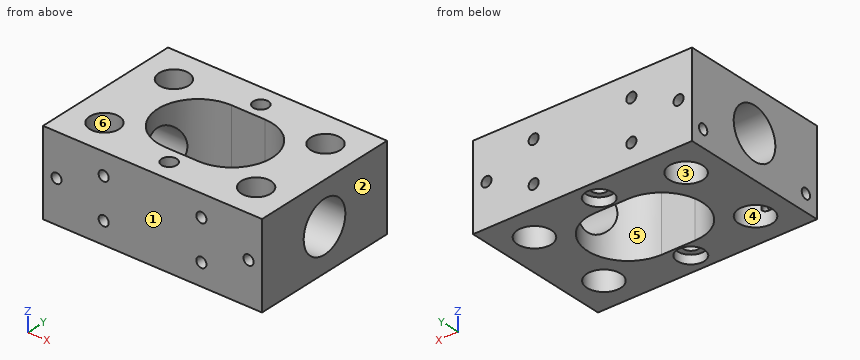
from build123d import *

# Parameters (mm, degrees)
SCHIZZO1_W                                           = 65
SCHIZZO1_H                                           = 45
ESTRUSIONE_ESTRUSIONE1_DEPTH                         = 25
SCHIZZO2_R                                           = 7.5
TAGLIO_ESTRUSIONE1_DEPTH                             = 83.915619759
FORO_LAMATO_PER_VITE_M4_A_TESTA_CILINDRI_D           = 4.5
FORO_LAMATO_PER_VITE_M4_A_TESTA_CILINDRI_CBORE_D     = 8
FORO_LAMATO_PER_VITE_M4_A_TESTA_CILINDRI_CBORE_DEPTH = 2.6
TAGLIO_ESTRUSIONE4_DEPTH                             = 83.915619759
SCHIZZO15_R                                          = 4.4
TAGLIO_ESTRUSIONE5_DEPTH                             = 6
SCHIZZO16_R                                          = 3
TAGLIO_ESTRUSIONE6_DEPTH                             = 82.308056285
SCHIZZO17_R                                          = 5
TAGLIO_ESTRUSIONE8_DEPTH                             = 10
FORO_3_0_3_1_D                                       = 3
FORO_3_0_3_1_DEPTH                                   = 12
FORO_3_0_3_1_TIP                                     = 0.901290929
FORO_3_0_3_2_D                                       = 3
FORO_3_0_3_2_DEPTH                                   = 12
FORO_3_0_3_2_TIP                                     = 0.901290929
FORO_3_0_3_3_D                                       = 3
FORO_3_0_3_3_DEPTH                                   = 12
FORO_3_0_3_3_TIP                                     = 0.901290929


with BuildPart() as part:
    # Schizzo1 → Estrusione-Estrusione1 (new body)
    with BuildSketch(Plane.XY):
        with Locations((32.5, 22.5)):
            Rectangle(SCHIZZO1_W, SCHIZZO1_H)
    extrude(amount=-ESTRUSIONE_ESTRUSIONE1_DEPTH)

    # Schizzo2 → Taglio-Estrusione1 (cut, through all)
    with BuildSketch(Plane.ZY):
        with Locations((-12.5, 22.5)):
            Circle(SCHIZZO2_R)
    extrude(amount=-TAGLIO_ESTRUSIONE1_DEPTH, mode=Mode.SUBTRACT)

    # Foro lamato per Vite M4 a testa cilindri (through all)
    with Locations(Plane(origin=(32.5, 39, -25), x_dir=(-1, 0, 0), z_dir=(0, 0, -1))):
        with Locations((0, 0), (0, -33)):
            CounterBoreHole(FORO_LAMATO_PER_VITE_M4_A_TESTA_CILINDRI_D / 2, FORO_LAMATO_PER_VITE_M4_A_TESTA_CILINDRI_CBORE_D / 2, FORO_LAMATO_PER_VITE_M4_A_TESTA_CILINDRI_CBORE_DEPTH)

    # Schizzo14 → Taglio-Estrusione4 (cut, through all)
    with BuildSketch(Plane.XY):
        with BuildLine():
            Line((37.5, 10.5), (27.5, 10.5))
            ThreePointArc((27.5, 10.5), (15.5, 22.5), (27.5, 34.5))
            Line((27.5, 34.5), (37.5, 34.5))
            ThreePointArc((37.5, 34.5), (49.5, 22.5), (37.5, 10.5))
        make_face()
    extrude(amount=-TAGLIO_ESTRUSIONE4_DEPTH, mode=Mode.SUBTRACT)

    # Schizzo15 → Taglio-Estrusione5 (cut)
    with BuildSketch(Plane.XY):
        with Locations((10, 10)):
            Circle(SCHIZZO15_R)
        with Locations(Location((55, 10, 0), (0, 0, 180))):
            Circle(SCHIZZO15_R)
        with Locations((55, 35)):
            Circle(SCHIZZO15_R)
        with Locations(Location((10, 35, 0), (0, 0, 180))):
            Circle(SCHIZZO15_R)
    extrude(amount=-TAGLIO_ESTRUSIONE5_DEPTH, mode=Mode.SUBTRACT)

    # Schizzo16 → Taglio-Estrusione6 (cut, through all)
    with BuildSketch(Plane.XY.offset(-6)):
        with Locations((10, 10)):
            Circle(SCHIZZO16_R)
        with Locations(Location((55, 10, 0), (0, 0, 180))):
            Circle(SCHIZZO16_R)
        with Locations((55, 35)):
            Circle(SCHIZZO16_R)
        with Locations(Location((10, 35, 0), (0, 0, 180))):
            Circle(SCHIZZO16_R)
    extrude(amount=-TAGLIO_ESTRUSIONE6_DEPTH, mode=Mode.SUBTRACT)

    # Schizzo17 → Taglio-Estrusione8 (cut)
    with BuildSketch(Plane(origin=(0, 0, -25), x_dir=(-1, 0, 0), z_dir=(0, 0, -1))):
        with Locations((-10, 10)):
            Circle(SCHIZZO17_R)
        with Locations(Location((-55, 10, 0), (0, 0, 180))):
            Circle(SCHIZZO17_R)
        with Locations((-55, 35)):
            Circle(SCHIZZO17_R)
        with Locations(Location((-10, 35, 0), (0, 0, 180))):
            Circle(SCHIZZO17_R)
    extrude(amount=-TAGLIO_ESTRUSIONE8_DEPTH, mode=Mode.SUBTRACT)

    # Foro _3.0 _3_-1
    with Locations(Plane(origin=(18, 45, -18.5), x_dir=(0, 0, 1), z_dir=(0, 1, 0))):
        with Locations((0, 0), (12, 0), (6, -14), (0, 29), (12, 29), (6, 43)):
            Hole(FORO_3_0_3_1_D / 2, depth=FORO_3_0_3_1_DEPTH)
            with Locations((0, 0, -(FORO_3_0_3_1_DEPTH + FORO_3_0_3_1_TIP / 2))):  # 118° drill point
                Cone(0, FORO_3_0_3_1_D / 2, FORO_3_0_3_1_TIP, mode=Mode.SUBTRACT)

    # Foro _3.0 _3_-2
    with Locations(Plane(origin=(18, 0, -6.5), x_dir=(0, 0, -1), z_dir=(0, -1, 0))):
        with Locations((0, 0), (6, -14), (12, 0), (0, 29), (12, 29), (6, 43)):
            Hole(FORO_3_0_3_2_D / 2, depth=FORO_3_0_3_2_DEPTH)
            with Locations((0, 0, -(FORO_3_0_3_2_DEPTH + FORO_3_0_3_2_TIP / 2))):  # 118° drill point
                Cone(0, FORO_3_0_3_2_D / 2, FORO_3_0_3_2_TIP, mode=Mode.SUBTRACT)

    # Foro _3.0 _3_-3
    with Locations(Plane(origin=(0, 41, -20), x_dir=(0, 0, -1), z_dir=(-1, 0, 0))):
        with Locations((0, 0), (0, 37)):
            Hole(FORO_3_0_3_3_D / 2, depth=FORO_3_0_3_3_DEPTH)
            with Locations((0, 0, -(FORO_3_0_3_3_DEPTH + FORO_3_0_3_3_TIP / 2))):  # 118° drill point
                Cone(0, FORO_3_0_3_3_D / 2, FORO_3_0_3_3_TIP, mode=Mode.SUBTRACT)


solid = part.part
Could you check a few things on this model? Use its own coordinates, in mm. Face numbers are marked on the shaded views. A direction names the side the tool comes from. Coordinates: 2 decimals unless noted, no trailing zeros. Order: outer loops, then holes, each group sorted by start corner. A loop starts at its lowest first (then second) coordinate and runs counter-clockwise, first axis right, second up. Notation, with made-up numbers: (77, 81) -> (99, 81) arc R20 cw to (99, 104) -> close; hole circle Ø7 at (38.25, -4.5). An arc over 180 degrees is marked (long way). One line per item, written item: value. Start each with the question number.
1) Which directions (+Z, -Z, +X, -X, +Y, -Y) give clear straight access to the entire face, cutting with the end or side of a thin tool? Please do the marked faces 4, 5 and 6.
2) If I drill on L1, parallel to Y at x = 55, z = -22.75; L2, parallel to Y at x = 10, z = -17; L3, parallel to Z at x = 47, y = 5, over which ranges is the centre line in solid material (lowest first)? Write a range as [from, to].
3) I'm going to push flat-ended pins straight in: pin 1 (4.5 mm diameter, centred on x = 57, y = 35.5, fed in from +Z); pin 2 (8 mm diameter, centred on y = 23.5, z = -12, fed in from +X). Where does each tip first touch, or does it pass through?
4) Imagine slicing it at A-A on x = 55. Count the separate pieces of the cut face and the enclosed holes in it, plus the area to 3 significant figures.
5) Imagine slicing it at B-B on x = 40. List the corners of the cut face in (y, z) for me.
6) We'd pull the mould along Y, two halves only. Please class the marked faces 1, 2 and 3: +Y half, -Y half, draft (parallel to the pull), parting line (faces both ways), or undercut.
Answer list:
1. face 4: -Z
1. face 5: +Z, -Z
1. face 6: +Z
2. L1: y = [0, 5], [15, 30], [40, 45]
2. L2: y = [0, 5], [15, 16.5], [28.5, 30], [40, 45]
2. L3: z = [-25, -20], [-17, -8], [-5, 0]
3. pin 1: stops at z = -6
3. pin 2: passes through
4. separate pieces: 3
4. enclosed holes: 1
4. area: 535 mm2
5. outline: (0, -25) -> (10.76, -25) -> (10.76, 0) -> (0, 0) -> close; (34.24, -25) -> (45, -25) -> (45, 0) -> (34.24, 0) -> close
6. face 1: -Y half
6. face 2: draft
6. face 3: undercut
